Answer from the drawing. Dimensions are ordinates in mm from the lowest x, y and z of the part. A direction names the side the tool comes from. Give positions to 0.01 mm unless a question says otherwise; leave off trailing zeros. Loops run counter-clockwise (first coordinate to the right, second up) from the corner with the lowest first, then second, coordinate; pieces in that order, holes last. Notation, with made-up numbers: (-17.75, 39.25) - (22.25, 39.25) arc R12 cw to (22.25, 49.25) - close; hole circle Ø7 at (16, 51). An arc over 180 degrees is marked (long way). Answer as CSV lines item,"result". Start each with the question number.
1) A cutting plane is placed at A-A (x = 124.5). Determine the outline of the cut face in (y, z).
2) A cutting plane is placed at C-C (y = 43). Determine the outline of the cut face in (x, z), and give its area (3 significant figures).
3) A cutting plane is placed at B-B (z = 3.5). Determine the outline of the cut face in (x, y), and give its area (3 significant figures).
4) For a pull along X with two mould halves and no side action, classify the marked faces 3, 4 and 5 as pulls with the +X half, pulls with the -X half, needs draft (parallel to the pull), parting line crosses it, or undercut.
5) Flat-ended cylindrical pins translate along their axes: pin 1 (2 mm diameter, centred on x = 124, y = 30, fed in from +Z); pin 2 (1 mm diameter, centred on x = 73, y = 61.5, fed in from -Z). Find the tip coordinate at first contact, or state that the pin passes through.
6) Find the intervals of material crossed by line 1 along Y through (x, z) = (29, 5.5); line 2 along X through (y, z) = (45, 6.25); line 3 along Z through (x, y) = (96, 65.5), in increasing order.
7) For the marked faces 1 and 2, determine the directions among +Z, -Z, +X, -X, +Y, -Y from which every point of the face is accessible in a straight line to the end or side of a thin tool.
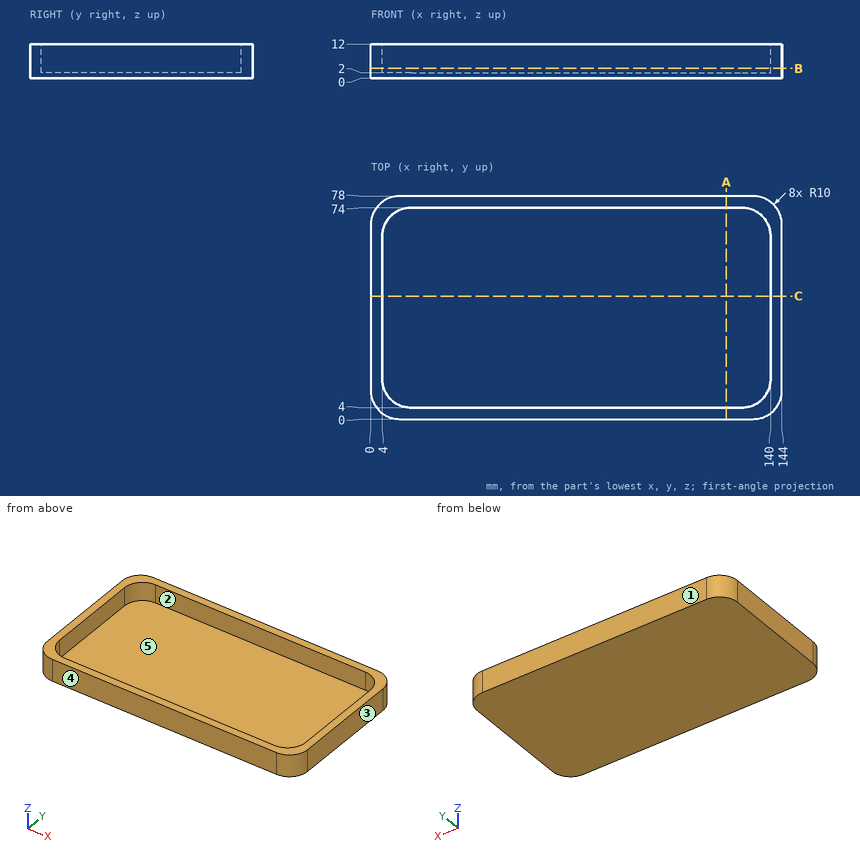
Ans:
1,outline,"(0, 0) - (78, 0) - (78, 12) - (74, 12) - (74, 2) - (4, 2) - (4, 12) - (0, 12) - close"
2,outline,"(0, 0) - (144, 0) - (144, 12) - (140, 12) - (140, 2) - (4, 2) - (4, 12) - (0, 12) - close"
2,area,"368 mm2"
3,outline,"(0, 10) arc R10 ccw to (10, 0) - (134, 0) arc R10 ccw to (144, 10) - (144, 68) arc R10 ccw to (134, 78) - (10, 78) arc R10 ccw to (0, 68) - close; hole (4, 14) arc R10 ccw to (14, 4) - (130, 4) arc R10 ccw to (140, 14) - (140, 64) arc R10 ccw to (130, 74) - (14, 74) arc R10 ccw to (4, 64) - close"
3,area,"1,710 mm2"
4,face 3,"pulls with the +X half"
4,face 4,"needs draft"
4,face 5,"undercut"
5,pin 1,"z = 2"
5,pin 2,"z = 0"
6,line 1,"0 to 4, 74 to 78"
6,line 2,"0 to 4, 140 to 144"
6,line 3,"0 to 2"
7,face 1,"+Z, -Z, +X, -X, +Y"
7,face 2,"+Z"
